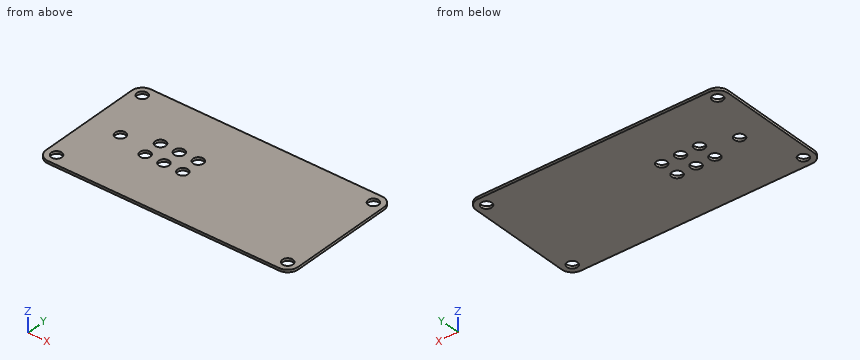
```python
from build123d import *

# Parameters (mm, degrees)
F1_DEPTH = 6
F2_D     = 25
F3_D     = 25
F4_D     = 25
F5_D     = 25


with BuildPart() as f1:
    # F0 (on Top) → F1 (new body)
    with BuildSketch(Plane.XY):
        with BuildLine():
            Line((-275, -150), (275, -150))
            ThreePointArc((275, -150), (292.6776695297, -142.6776695297), (300, -125))
            Line((300, -125), (300, 125))
            ThreePointArc((300, 125), (292.6776695297, 142.6776695297), (275, 150))
            Line((275, 150), (-275, 150))
            ThreePointArc((-275, 150), (-292.6776695297, 142.6776695297), (-300, 125))
            Line((-300, 125), (-300, -125))
            ThreePointArc((-300, -125), (-292.6776695297, -142.6776695297), (-275, -150))
        make_face()
    extrude(amount=F1_DEPTH)

    # F2 (through all)
    with Locations(Plane(origin=(0, 0, 0), x_dir=(1, 0, 0), z_dir=(0, 0, -1))):
        with Locations((-275, 125)):
            Hole(F2_D / 2)

    # F3 (through all)
    with Locations(Plane(origin=(0, 0, 0), x_dir=(1, 0, 0), z_dir=(0, 0, -1))):
        with Locations((-275, -125), (275, 125)):
            Hole(F3_D / 2)

    # F4 (through all)
    with Locations(Plane(origin=(0, 0, 0), x_dir=(1, 0, 0), z_dir=(0, 0, -1))):
        with Locations((275, -125)):
            Hole(F4_D / 2)

    # F5 (through all)
    with Locations(Plane(origin=(0, 0, 0), x_dir=(1, 0, 0), z_dir=(0, 0, -1))):
        with Locations((-150, -24.8980756774), (-105, -24.8980756774), (-60, -24.8980756774), (-60, 20.1019243226), (-105, 20.1019243226), (-150, 20.1019243226), (-225, 0)):
            Hole(F5_D / 2)


solid = f1.part
```
Work out the finished part from the listing and answer in its coordinate system (mm). Give positions to 0.01 mm unless a question says otherwise; leave off trailing zeros. Loops run counter-clockwise (first coordinate to the right, second up) from the corner with the lowest first, then second, coordinate; pieces in that order, holes last. Notation, with made-up numbers: (87.5, 68) -> (136.5, 68) arc R12 ccw to (136.5, 86) -> close; hole circle Ø11 at (4, -15.5). An arc over 180 degrees is marked (long way). One line per question, with ' | ' between items. Start each with the question number.
1) Section D-D, the plane x = -54 is taken. Determine the outline of the cut face in (y, z), then the cut area to 3 significant figures.
2) Section B-B, the plane x = -150 is taken. Determine the outline of the cut face in (y, z).
3) Straight lines are drawn through the part: L1, parallel to Y at x = -275, z = 4.45; L2, parallel to X at y = -125, z = 1.35; L3, parallel to Y at x = -61, z = 3.5. For each, find the intervals that lie inside material, in ascending order.
4) Section C-C, the plane z = 1.9 is taken. State how many separate pieces and enclosed holes the cut face has, then the cut area to 3 significant figures.
5) Section A-A, the plane x = -225 is taken. Determine the outline of the cut face in (y, z).
Resolved:
1) outline: (-150, 0) -> (-31.07, 0) -> (-31.07, 6) -> (-150, 6) -> close; (-9.14, 0) -> (13.93, 0) -> (13.93, 6) -> (-9.14, 6) -> close; (35.86, 0) -> (150, 0) -> (150, 6) -> (35.86, 6) -> close | area: 1,540 mm2
2) outline: (-150, 0) -> (-32.6, 0) -> (-32.6, 6) -> (-150, 6) -> close; (-7.6, 0) -> (12.4, 0) -> (12.4, 6) -> (-7.6, 6) -> close; (37.4, 0) -> (150, 0) -> (150, 6) -> (37.4, 6) -> close
3) L1: -150 to -137.5, -112.5 to 112.5, 137.5 to 150 | L2: -300 to -287.5, -262.5 to 262.5, 287.5 to 300 | L3: -150 to -32.56, -7.64 to 12.44, 37.36 to 150
4) separate pieces: 1 | enclosed holes: 11 | area: 174,000 mm2
5) outline: (-150, 0) -> (-12.5, 0) -> (-12.5, 6) -> (-150, 6) -> close; (12.5, 0) -> (150, 0) -> (150, 6) -> (12.5, 6) -> close
